from build123d import *

# Parameters (mm, degrees)
SKETCH1_R               = 24.95
BOSS_EXTRUDE1_DEPTH     = 332.5
CUT_EXTRUDE1_DEPTH      = 335.366946632
CUT_EXTRUDE1_DEPTH_BACK = 335.366946632
SKETCH2_R               = 10.05
CUT_EXTRUDE2_DEPTH      = 337.253855116
SKETCH5_OUTSIDE_W       = 185.646
SKETCH5_OUTSIDE_H       = 185.646
SKETCH5_OUTSIDE_R       = 24.61
CUT_EXTRUDE4_DEPTH      = 200
SKETCH7_OUTSIDE_W       = 185.646
SKETCH7_OUTSIDE_H       = 185.646
SKETCH7_OUTSIDE_R       = 22.3
CUT_EXTRUDE6_DEPTH      = 50
CUT_EXTRUDE7_DEPTH      = 7
CIRPATTERN1_COUNT       = 4


with BuildPart() as part:
    # Sketch1 → Boss-Extrude1 (new, symmetric)
    with BuildSketch(Plane.XY):
        Circle(SKETCH1_R)
    extrude(amount=BOSS_EXTRUDE1_DEPTH, both=True)

    # Sketch2 → Cut-Extrude1 (cut, two sides: drawn at the far end of the back side and taken through both)
    with BuildSketch(Plane(origin=(0, 0, 0), x_dir=(0, 0, -1), z_dir=(1, 0, 0)).offset(-CUT_EXTRUDE1_DEPTH_BACK)):
        with Locations(Location((192.5, 0, 0), (0, 0, 180))):
            Circle(SKETCH2_R)
        with Locations(Location((292.5, 0, 0), (0, 0, 180))):
            Circle(SKETCH2_R)
    extrude(amount=CUT_EXTRUDE1_DEPTH + CUT_EXTRUDE1_DEPTH_BACK, mode=Mode.SUBTRACT)

    # Sketch3 → Cut-Extrude2 (cut, through all)
    with BuildSketch(Plane(origin=(-18.5, 0, 0), x_dir=(0, 0, -1), z_dir=(1, 0, 0))):
        with BuildLine():
            Line((-212.5, -7), (-170.5, -7))
            ThreePointArc((-170.5, -7), (-163.5, 0), (-170.5, 7))
            Line((-170.5, 7), (-212.5, 7))
            ThreePointArc((-212.5, 7), (-219.5, 0), (-212.5, -7))
        make_face()
    extrude(amount=-CUT_EXTRUDE2_DEPTH, mode=Mode.SUBTRACT)

    # Sketch5 outside → Cut-Extrude4 (cut)
    with BuildSketch(Plane(origin=(0, 0, -332.5), x_dir=(-1, 0, 0), z_dir=(0, 0, -1))):
        Rectangle(SKETCH5_OUTSIDE_W, SKETCH5_OUTSIDE_H)
        Circle(SKETCH5_OUTSIDE_R, mode=Mode.SUBTRACT)
    extrude(amount=-CUT_EXTRUDE4_DEPTH, mode=Mode.SUBTRACT)

    # Sketch7 outside → Cut-Extrude6 (cut)
    with BuildSketch(Plane.XY.offset(332.5)):
        Rectangle(SKETCH7_OUTSIDE_W, SKETCH7_OUTSIDE_H)
        Circle(SKETCH7_OUTSIDE_R, mode=Mode.SUBTRACT)
    extrude(amount=-CUT_EXTRUDE6_DEPTH, mode=Mode.SUBTRACT)

    # Sketch8 → Cut-Extrude7 (cut)
    with BuildSketch(Plane(origin=(3.872354362, 21.961212892, 0), x_dir=(0, 0, 1), z_dir=(0.1736481776669241, 0.9848077530122091, 0))):
        with BuildLine():
            Line((292.5, 7), (332.5, 7))
            ThreePointArc((332.5, 7), (339.5, 0), (332.5, -7))
            Line((332.5, -7), (292.5, -7))
            ThreePointArc((292.5, -7), (285.5, 0), (292.5, 7))
        make_face()
    cut_extrude7 = extrude(amount=-CUT_EXTRUDE7_DEPTH, mode=Mode.SUBTRACT)

    # CirPattern1: Cut-Extrude7 ×4 about axis
    cirpattern1_axis = Axis((0, 0, 0), (0, 0, 1))
    for i in range(1, CIRPATTERN1_COUNT):
        add(cut_extrude7.rotate(cirpattern1_axis, i * 360 / CIRPATTERN1_COUNT), mode=Mode.SUBTRACT)


solid = part.part
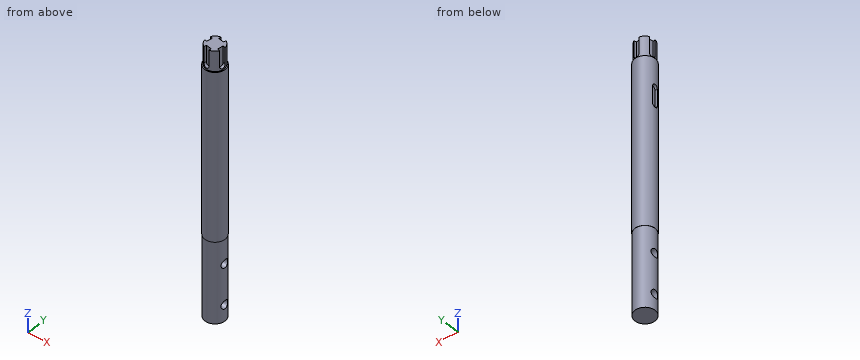
The listing builds one solid part. Answer for the finished solid, in the listing's coordinates (mm). Round coordinates to 2 decimals unless told otherwise and drop trailing zeros. Order: outer loops, then holes, each group sorted by start corner. A loop starts at its lowest first (then second) coordinate and runs counter-clockwise, first axis right, second up. Notation, with made-up numbers: M 14,54.5 L 72,54.5 A22 cw 72,71.5 Z; hole C 20.25,2 d2. An arc over 180 degrees is marked long. Answer in a Markdown table with one row per item. Add a question column.
1) Consider line 1 along Y through (x, z) = (1, -192); line 2 along Y through (x, z) = (-19, -122.5); line 3 along Y through (x, z) = (-6, -192). Determine where each line is inside the solid, lowest interval first. Write a range as from..to.
2) Flat-ended cylindrical pins translate along their axes: pin 1 Ø1.6 at (x, z) = (-20, 187) entering from +Y; pin 2 Ø4 at (y, z) = (-2.5, 181) entering from -X; pin 3 Ø2 at (x, z) = (-4, -164.5) entering from +Y. Find the tip coordinate at first contact, or state that the pin passes through.
3) The part is cut by section B-B on z = -55. Determine the outline of the cut face in (x, y).
4) The part is cut by section A-A on z = -291. Determine the outline of the cut face in (x, y).
Findings below:
| question | item | result |
|---|---|---|
| 1 | line 1 | y = -24.59..-10.04, 10.04..24.59 |
| 1 | line 2 | y = -16.17..16.17 |
| 1 | line 3 | y = -23.87..-10.04, 10.04..23.87 |
| 2 | pin 1 | stops at y = 15.93 |
| 2 | pin 2 | stops at x = -18.5 |
| 2 | pin 3 | stops at y = 24.43 |
| 3 | outline | C 0,0 d49.9 |
| 4 | outline | M -22.51,-9.94 A24.61 ccw 22.51,-9.94 Z; M -22.51,9.94 L 22.51,9.94 A24.61 ccw Z |
